Design review of the part built by this model. Coordinates are the model's own, in mm. Face numbers are marked on the shaded views. A direction names the side the tool comes from. Give positions to 0.01 mm unless a question says otherwise; leave off trailing zeros. Write each loop counter-clockwise with the first axis right and the second up, starting at its lowest first coordinate (ties: lowest second). Pieces come first, ordered by that corner, then holes. Notation, with made-up numbers: M -9.75,49 L 7.25,49 A25 ccw 7.25,73 Z; hole C 35,-9 d11. An arc over 180 degrees is marked long. Use a Markdown table: item, result. Add a question column.
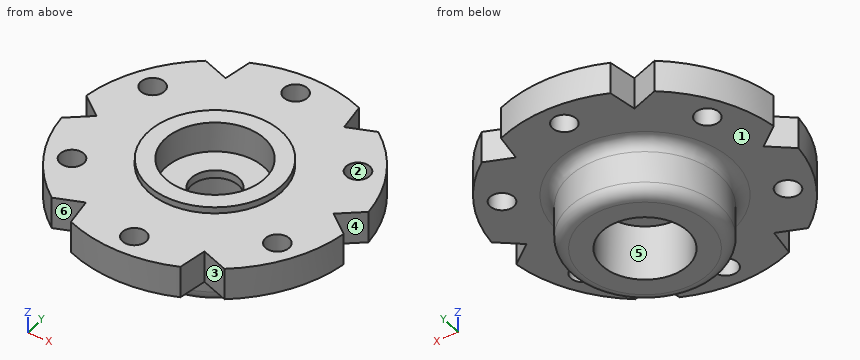
```python
from build123d import *

# Parameters (mm, degrees)
SKETCH1_R           = 1.5
SKETCH1_R_2         = 0.75
BOSS_EXTRUDE1_DEPTH = 2
SKETCH2_R           = 4.75
SKETCH2_R_2         = 2.7
BOSS_EXTRUDE2_DEPTH = 3.5
SKETCH3_R           = 4.2
SKETCH3_R_2         = 3.125
BOSS_EXTRUDE3_DEPTH = 0.4
SKETCH4_R           = 3.125
CUT_EXTRUDE1_DEPTH  = 1.5
FILLET1_R           = 0.75
SKETCH5_OUTSIDE_W   = 39.274
SKETCH5_OUTSIDE_H   = 42.892
SKETCH5_OUTSIDE_R   = 9
CUT_EXTRUDE2_DEPTH  = 6.5


with BuildPart() as part:
    # Sketch1 → Boss-Extrude1 (new body)
    with BuildSketch(Plane.XY):
        with BuildLine():
            Line((-2.567552709, 13.90947904), (-3.75, 6.495190528))
            Line((-3.75, 6.495190528), (-10.762185848, 9.178305392))
            ThreePointArc((-10.762185848, 9.178305392), (-13.943009001, 8.05), (-13.329738557, 4.731173648))
            Line((-13.329738557, 4.731173648), (-7.5, 0))
            Line((-7.5, 0), (-13.329738557, -4.731173648))
            ThreePointArc((-13.329738557, -4.731173648), (-13.943009001, -8.05), (-10.762185848, -9.178305392))
            Line((-10.762185848, -9.178305392), (-3.75, -6.495190528))
            Line((-3.75, -6.495190528), (-2.567552709, -13.90947904))
            ThreePointArc((-2.567552709, -13.90947904), (0, -16.1), (2.567552709, -13.90947904))
            Line((2.567552709, -13.90947904), (3.75, -6.495190528))
            Line((3.75, -6.495190528), (10.762185848, -9.178305392))
            ThreePointArc((10.762185848, -9.178305392), (13.943009001, -8.05), (13.329738557, -4.731173648))
            Line((13.329738557, -4.731173648), (7.5, 0))
            Line((7.5, 0), (13.329738557, 4.731173648))
            ThreePointArc((13.329738557, 4.731173648), (13.943009001, 8.05), (10.762185848, 9.178305392))
            Line((10.762185848, 9.178305392), (3.75, 6.495190528))
            Line((3.75, 6.495190528), (2.567552709, 13.90947904))
            ThreePointArc((2.567552709, 13.90947904), (0, 16.1), (-2.567552709, 13.90947904))
        make_face()
        Circle(SKETCH1_R, mode=Mode.SUBTRACT)
        with Locations((0, 13.5)):
            Circle(SKETCH1_R_2, mode=Mode.SUBTRACT)
        with Locations((0, 10.5)):
            Circle(SKETCH1_R_2, mode=Mode.SUBTRACT)
        with Locations((0, 7.5)):
            Circle(SKETCH1_R_2, mode=Mode.SUBTRACT)
        with Locations((6.495190528, 3.75)):
            Circle(SKETCH1_R_2, mode=Mode.SUBTRACT)
        with Locations((9.09326674, 5.25)):
            Circle(SKETCH1_R_2, mode=Mode.SUBTRACT)
        with Locations((11.691342951, 6.75)):
            Circle(SKETCH1_R_2, mode=Mode.SUBTRACT)
        with Locations((6.495190528, -3.75)):
            Circle(SKETCH1_R_2, mode=Mode.SUBTRACT)
        with Locations((9.09326674, -5.25)):
            Circle(SKETCH1_R_2, mode=Mode.SUBTRACT)
        with Locations((11.691342951, -6.75)):
            Circle(SKETCH1_R_2, mode=Mode.SUBTRACT)
        with Locations((0, -7.5)):
            Circle(SKETCH1_R_2, mode=Mode.SUBTRACT)
        with Locations((0, -10.5)):
            Circle(SKETCH1_R_2, mode=Mode.SUBTRACT)
        with Locations((0, -13.5)):
            Circle(SKETCH1_R_2, mode=Mode.SUBTRACT)
        with Locations((-6.495190528, -3.75)):
            Circle(SKETCH1_R_2, mode=Mode.SUBTRACT)
        with Locations((-9.09326674, -5.25)):
            Circle(SKETCH1_R_2, mode=Mode.SUBTRACT)
        with Locations((-11.691342951, -6.75)):
            Circle(SKETCH1_R_2, mode=Mode.SUBTRACT)
        with Locations((-6.495190528, 3.75)):
            Circle(SKETCH1_R_2, mode=Mode.SUBTRACT)
        with Locations((-9.09326674, 5.25)):
            Circle(SKETCH1_R_2, mode=Mode.SUBTRACT)
        with Locations((-11.691342951, 6.75)):
            Circle(SKETCH1_R_2, mode=Mode.SUBTRACT)
    extrude(amount=BOSS_EXTRUDE1_DEPTH)

    # Sketch2 → Boss-Extrude2 (add)
    with BuildSketch(Plane(origin=(0, 0, 0), x_dir=(-1, 0, 0), z_dir=(0, 0, -1))):
        Circle(SKETCH2_R)
        Circle(SKETCH2_R_2, mode=Mode.SUBTRACT)
    extrude(amount=BOSS_EXTRUDE2_DEPTH)

    # Sketch3 → Boss-Extrude3 (add)
    with BuildSketch(Plane.XY.offset(2)):
        Circle(SKETCH3_R)
        Circle(SKETCH3_R_2, mode=Mode.SUBTRACT)
    extrude(amount=BOSS_EXTRUDE3_DEPTH)

    # Sketch4 → Cut-Extrude1 (cut)
    with BuildSketch(Plane.XY.offset(2)):
        Circle(SKETCH4_R)
    extrude(amount=-CUT_EXTRUDE1_DEPTH, mode=Mode.SUBTRACT)

    # Fillet1
    fillet1_edges = [part.edges().sort_by_distance(p)[0] for p in [
        (4.75, 0, 0),
        (4.75, 0, -3.5),
    ]]
    fillet(fillet1_edges, radius=FILLET1_R)

    # Sketch5 outside → Cut-Extrude2 (cut, through all)
    with BuildSketch(Plane.XY.offset(2)):
        Rectangle(SKETCH5_OUTSIDE_W, SKETCH5_OUTSIDE_H)
        Circle(SKETCH5_OUTSIDE_R, mode=Mode.SUBTRACT)
    extrude(amount=-CUT_EXTRUDE2_DEPTH, mode=Mode.SUBTRACT)


solid = part.part
```
(1) Machinability: for the marked faces 4, 5 and 6, which of the approach directions +Z, -Z, +X, -X, +Y, -Y give a long, thin tool a straight path to every point of the face, cutting with its end or side? Answer none if there is none.
(2) Add section B-B on z = 1.7. Give the boundary of the cut face in (x, y) (3 decimals).
(3) The part is to be moulded in two halves that separate along Y. For the marked faces 1, 2 and 3, say which applies: released by +Y, released by -Y, zero draft, split by the parting line, or undercut.
(4) For pin 1 (1.7 mm diameter, centred on x = -6.5, y = 3.75, fed in from -Z); pin 2 (1.7 mm diameter, centred on x = 0, y = 7.5, fed in from +Z), all flat-tipped, find the tip position at first contact; note any pin that passes through.
(5) Add section A-A on y = -7.5. Give the boundary of the cut face in (x, z).
(6) Add section C-C on x = 0. Give the number of separate pieces and of enclosed holes in the cut face, then the cut area to 3 significant figures.
(7) Add section D-D on z = -1.6. Give the boundary of the cut face in (x, y), then the cut area to 3 significant figures.
(8) Wall thickness on L1, parallel to Y at x = 0, z = 0.45; L2, parallel to Z at x = -1.75, y = -0.25; L3, parallel to Y at x = 0.75, z = -1.7: over which ranges is each line inside the solid? List them lowest first.
From the geometry:
| question | item | result |
|---|---|---|
| 1 | face 4 | +Z, -Z, +X |
| 1 | face 5 | -Z |
| 1 | face 6 | +Z, -Z, -Y |
| 2 | outline | M -8.925,-1.157 A9 ccw -5.464,-7.151 L -3.75,-6.495 L -3.461,-8.308 A9 ccw 3.461,-8.308 L 3.75,-6.495 L 5.464,-7.151 A9 ccw 8.925,-1.157 L 7.5,0 L 8.925,1.157 A9 ccw 5.464,7.151 L 3.75,6.495 L 3.461,8.308 A9 ccw -3.461,8.308 L -3.75,6.495 L -5.464,7.151 A9 ccw -8.925,1.157 L -7.5,0 Z; hole C -6.495,-3.75 d1.5; hole C -6.495,3.75 d1.5; hole C 0,0 d6.25; hole C 0,-7.5 d1.5; hole C 0,7.5 d1.5; hole C 6.495,-3.75 d1.5; hole C 6.495,3.75 d1.5 |
| 3 | face 1 | zero draft |
| 3 | face 2 | undercut |
| 3 | face 3 | released by -Y |
| 4 | pin 1 | stops at z = 0 |
| 4 | pin 2 | stops at z = 2 |
| 5 | outline | M -3.59,0 L -0.75,0 L -0.75,2 L -3.59,2 Z; M 0.75,0 L 3.59,0 L 3.59,2 L 0.75,2 Z |
| 6 | separate pieces | 4 |
| 6 | enclosed holes | 0 |
| 6 | area | 34.3 mm^2 |
| 7 | outline | C 0,0 d9.5; hole C 0,0 d5.4 |
| 7 | area | 48.0 mm^2 |
| 8 | L1 | y = -9 to -8.25, -6.75 to -1.5, 1.5 to 6.75, 8.25 to 9 |
| 8 | L2 | z = 0 to 0.5 |
| 8 | L3 | y = -4.69 to -2.59, 2.59 to 4.69 |
